Autodesk Inventor part; units mm, degrees
ref_plane "工作平面2" through (10, 0, 0) normal (-1, 0, 0) x (0, 0, 1)
ref_plane "工作平面4" through (0, 0, 20) normal (0, 0, 1) x (1, 0, 0)
ref_plane "YZ Plane" through (0, 0, 0) normal (1, 0, 0) x (0, 1, 0)
sketch "草圖1" plane through (0, 0, 0) normal (0, 1, 0) x (-1, 0, 0)
  line L0 (0, 0) -> (-60, 0)
  line L1 (-60, 0) -> (-60, 40)
  line L2 (-60, 40) -> (0, 40)
  line L3 (0, 40) -> (0, 0)
  dimension "d0" = 40
  dimension "d1" = 60
extrude "擠出1" add sketch "草圖1" along normal blind 40
sketch "草圖3" plane through (60, 0, 40) normal (1, 0, 0) x (0, 0, -1)
  line L0 (40, 40) -> (40, 0)
  line L1 (40, 0) -> (0, 0) construction
  line L2 (0, 0) -> (0, 40) construction
  line L3 (0, 40) -> (40, 40) construction
  line L4 (40, 40) -> (0, 40) construction
  line L5 (40, 0) -> (40, 40)
  line L6 (40, 10) -> (20, 30)
  line L7 (20, 30) -> (40, 40)
  dimension "d14" = 30
  dimension "d15" = 20
  dimension "d16" = 10
ref_plane "工作平面2" through (10, 0, 0) normal (-1, 0, 0) x (0, 0, 1)
sketch "草圖7" plane through (10, 0, 0) normal (-1, 0, 0) x (0, 0, 1)
  line L0 (0, 0) -> (0, 40) construction
  line L1 (0, 40) -> (40, 40) construction
  line L2 (40, 40) -> (40, 0) construction
  line L3 (40, 0) -> (0, 0) construction
loft "斷面混成2" cut profiles "草圖3" section 2 point at (10, 40, 0)
ref_plane "工作平面4" through (0, 0, 20) normal (0, 0, 1) x (1, 0, 0)
mirror "鏡射2" about plane through (0, 0, 20) normal (0, 0, 1) of "斷面混成2"
sketch "草圖18" plane through (60, 0, 0) normal (0, 0, -1) x (-1, 0, 0)
  line L0 (60, 40) -> (60, 0)
  line L1 (60, 0) -> (0, 0)
  line L2 (0, 0) -> (0, 10)
  line L3 (0, 10) -> (50, 40)
  line L4 (50, 40) -> (60, 40)
  line L5 (50, 40) -> (0, 40)
  line L6 (60, 40) -> (50, 40)
  line L7 (0, 30) -> (50, 40)
  line L8 (50, 40) -> (0, 30)
  line L9 (0, 30) -> (0, 40)
  line L10 (50, 40) -> (0, 40)
  line L11 (0, 40) -> (50, 40)
extrude "擠出2" cut sketch "草圖18" against normal blind 45 contours L7 L9 L5
properties part number "16" material "鋼、碳鋼"
Geometry check sheet. Reference: the model listing, model coordinates, mm. Round coordinates to 2 decimals unless told otherwise and drop trailing zeros. Loops run counter-clockwise (first coordinate to the right, second up) from the corner with the lowest first, then second, coordinate; pieces in that order, holes last. Notation, with made-up numbers: (-25, 52.5) - (15, 52.5) arc R4 ccw to (15, 57.5) - close; hole circle Ø4 at (-14, -31.5). An arc over 180 degrees is marked (long way). Use a Markdown table: item, result.
Q1. Cross-section at A-A on y = 28. Record the cut outline in (x, z).
Solutions:
| item | result |
|---|---|
| outline | (0, 0) - (30, 0) - (60, 18) - (60, 22) - (30, 40) - (0, 40) - close |
Q2. Cross-section at B-B on x = 46. Record the cut outline in (y, z), plus the area to 3 significant figures.
Solutions:
| item | result |
|---|---|
| outline | (0, 0) - (18.4, 0) - (32.8, 14.4) - (32.8, 25.6) - (18.4, 40) - (0, 40) - close |
| area | 1,100 mm2 |
Q3. Material ranges on line 1 (Y direction, x = 13, z = 2); line 2 (Y direction, x = 45, z = 17.5); line 3 (X direction, y = 30, z = 34), recorded low to high.
Solutions:
| item | result |
|---|---|
| line 1 | y = 0 to 39.4 |
| line 2 | y = 0 to 33 |
| line 3 | x = 0 to 36.67 |
Q4. Go/stop test with flat-tipped pins: P1, Ø6, axis at y = 28, z = 13.5, coming from the -X side; P2, Ø6, axis at y = 26, z = 9.5, coming from the +X side; P3, Ø2, axis at y = 27.5, z = 34.5, coming from the +X side; P4, Ø2, axis at y = 28, z = 23.5, coming from the +X side. Record where each tip stops, or that it passes through.
Solutions:
| item | result |
|---|---|
| P1 | stops at x = 0 |
| P2 | stops at x = 56.24 |
| P3 | stops at x = 42.36 |
| P4 | stops at x = 59.86 |
